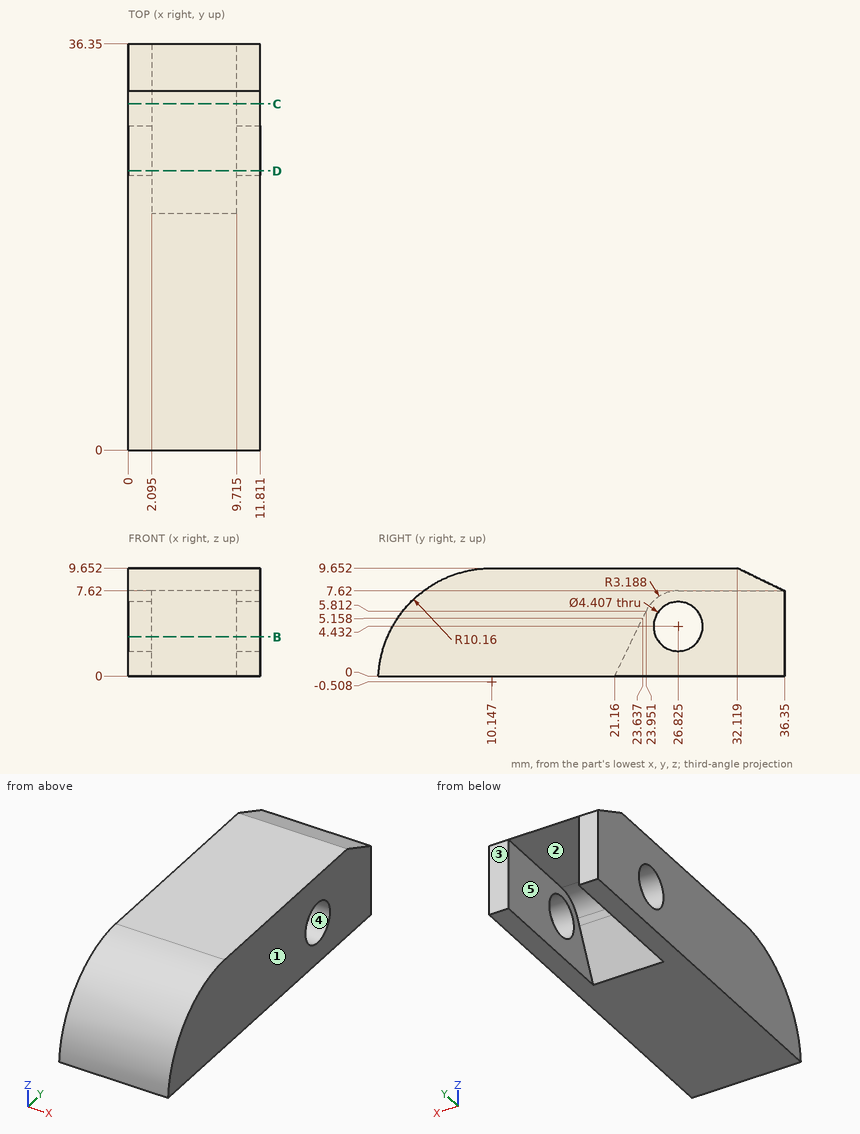
Geometry check sheet. Reference: drawing and pictorial views, mm from the part's lowest x, y, z. A direction names the side the tool comes from. Round coordinates to 2 decimals unless told otherwise and drop trailing zeros. Loops run counter-clockwise (first coordinate to the right, second up) from the corner with the lowest first, then second, coordinate; pieces in that order, holes last. Notation, with made-up numbers: (46, 39) -> (79, 39) arc R19 ccw to (79, 64) -> close; hole circle Ø7 at (-7.5, 53.5). An arc over 180 degrees is marked (long way). Use a Markdown table: item, result.
(1) Sectioned sample at C-C (y = 31). Enter the section's corners in (x, z) (1 decimal).
Calculated:
| item | result |
|---|---|
| outline | (0, 0) -> (2.1, 0) -> (2.1, 7.6) -> (9.7, 7.6) -> (9.7, 0) -> (11.8, 0) -> (11.8, 9.7) -> (0, 9.7) -> close |
(2) Set-up check for the marked faces 4 and 5: record each of +Z, -Z, +X, -X, +Y, -Y from which the full face is reachable in a straight line by a thin tool's end or side.
Calculated:
| item | result |
|---|---|
| face 4 | +X, -X |
| face 5 | -Z, +Y |
(3) Scan lines: probe 1 along X at (y, z) = (31, 4.75) (1 decimal); probe 2 along Z at (x, y) = (3.25, 30); probe 3 along Y at (x, z) = (7.5, 6.5). Record each from-to range of solid material in increasing order.
Calculated:
| item | result |
|---|---|
| probe 1 | 0 to 2.1, 9.7 to 11.8 |
| probe 2 | 7.62 to 9.65 |
| probe 3 | 2.79 to 24.4 |
(4) Go/stop test with a flat-tipped pin: P1, Ø3.5, axis at y = 26.82, z = 4.43, coming from the +X side. Record where the tip stops, or that it passes through.
Calculated:
| item | result |
|---|---|
| P1 | through |
(5) Sectioned sample at D-D (y = 25). Enter the section's corners in (x, z) (1 decimal).
Calculated:
| item | result |
|---|---|
| outline | (0, 0) -> (2.1, 0) -> (2.1, 3.2) -> (0, 3.2) -> close; (0, 5.7) -> (2.1, 5.7) -> (2.1, 7) -> (9.7, 7) -> (9.7, 5.7) -> (11.8, 5.7) -> (11.8, 9.7) -> (0, 9.7) -> close; (9.7, 0) -> (11.8, 0) -> (11.8, 3.2) -> (9.7, 3.2) -> close |
(6) Sectioned sample at B-B (z = 3.5). Give the number of separate pieces and of enclosed holes in the cut face, then the cut area to 3 significant figures.
Calculated:
| item | result |
|---|---|
| separate pieces | 3 |
| enclosed holes | 0 |
| area | 300 mm² |
(7) Mould release check, pull along X, two halves, no side actions. Record for the marked faces 1, 2 and 3: released by +X, released by -X, zero draft, split by the parting line, or undercut.
Calculated:
| item | result |
|---|---|
| face 1 | released by +X |
| face 2 | undercut |
| face 3 | zero draft |
